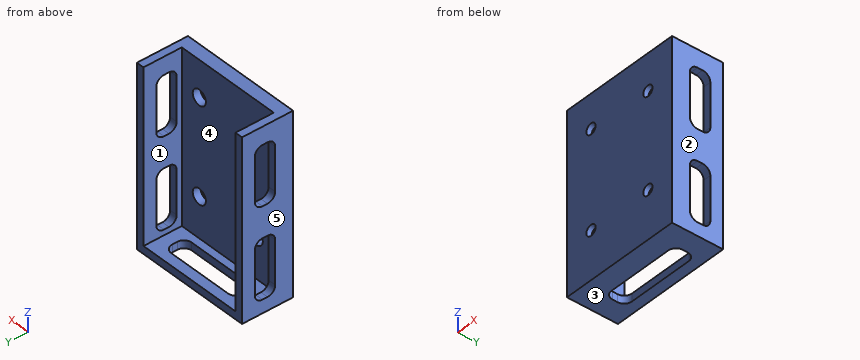
```python
from build123d import *

# Parameters (mm, degrees)
EXTRUDE_1_DEPTH     = 70
SKETCH_2_W          = 3
SKETCH_2_H          = 15
EXTRUDE_2_DEPTH     = 70
EXTRUDE_3_REACH     = 86.588
SKETCH_3_W          = 3
SKETCH_3_H          = 15
CUT_EXTRUDE_1_DEPTH = 87.22126548
CUT_EXTRUDE_2_DEPTH = 73.767483267
SKETCH_6_R          = 3
CUT_EXTRUDE_3_DEPTH = 3
SKETCH_7_R          = 2.1
CUT_EXTRUDE_4_DEPTH = 77.157731059


with BuildPart() as part:
    # 草图1 → 凸台-拉伸1 (new body)
    with BuildSketch(Plane.XY):
        Polygon((0, -15.16926567), (-24, -15.16926567), (-24, -10.16926567), (0, -10.16926567), (24, -10.16926567), (24, -15.16926567), align=None)
    extrude(amount=EXTRUDE_1_DEPTH)

    # 草图2 → 凸台-拉伸2 (add)
    with BuildSketch(Plane(origin=(0, 0, 0), x_dir=(-1, 0, 0), z_dir=(0, 0, -1))):
        with Locations((-22.5, -2.66926567)):
            Rectangle(SKETCH_2_W, SKETCH_2_H)
        with Locations((22.5, -2.66926567)):
            Rectangle(SKETCH_2_W, SKETCH_2_H)
    extrude(amount=-EXTRUDE_2_DEPTH)

    # 草图3 → 凸台-拉伸3 (add, up to next)
    with BuildSketch(Plane.ZY.offset(-21), mode=Mode.PRIVATE) as extrude_3_sk1:
        with Locations((1.5, -2.66926567)):
            Rectangle(SKETCH_3_W, SKETCH_3_H)
    extrude_3_tool1 = extrude(extrude_3_sk1.sketch, amount=EXTRUDE_3_REACH, mode=Mode.PRIVATE) - part.part
    add(extrude_3_tool1.solids().sort_by_distance((21, -2.669266, 1.5))[0])

    # 草图4 → 切除-拉伸1 (cut, through all)
    with BuildSketch(Plane.ZY.offset(24)):
        with BuildLine():
            Line((5.140274164, -3.16926567), (5.140274164, -5.16926567))
            ThreePointArc((5.140274164, -5.16926567), (6.018953821, -7.290586014), (8.140274164, -8.16926567))
            Line((8.140274164, -8.16926567), (25.140274164, -8.16926567))
            ThreePointArc((25.140274164, -8.16926567), (27.261594508, -7.290586014), (28.140274164, -5.16926567))
            Line((28.140274164, -5.16926567), (28.140274164, -3.16926567))
            ThreePointArc((28.140274164, -3.16926567), (27.261594508, -1.047945327), (25.140274164, -0.16926567))
            Line((25.140274164, -0.16926567), (8.140274164, -0.16926567))
            ThreePointArc((8.140274164, -0.16926567), (6.018953821, -1.047945327), (5.140274164, -3.16926567))
        make_face()
        with BuildLine():
            Line((40.140274164, -3.16926567), (40.140274164, -5.16926567))
            ThreePointArc((40.140274164, -5.16926567), (41.018953821, -7.290586014), (43.140274164, -8.16926567))
            Line((43.140274164, -8.16926567), (60.140274164, -8.16926567))
            ThreePointArc((60.140274164, -8.16926567), (62.261594508, -7.290586014), (63.140274164, -5.16926567))
            Line((63.140274164, -5.16926567), (63.140274164, -3.16926567))
            ThreePointArc((63.140274164, -3.16926567), (62.261594508, -1.047945327), (60.140274164, -0.16926567))
            Line((60.140274164, -0.16926567), (43.140274164, -0.16926567))
            ThreePointArc((43.140274164, -0.16926567), (41.018953821, -1.047945327), (40.140274164, -3.16926567))
        make_face()
    extrude(amount=-CUT_EXTRUDE_1_DEPTH, mode=Mode.SUBTRACT)

    # 草图5 → 切除-拉伸2 (cut, through all)
    with BuildSketch(Plane.XY.offset(3)):
        with BuildLine():
            Line((-13, 0.83073433), (13, 0.83073433))
            ThreePointArc((13, 0.83073433), (15.121320344, -0.047945327), (16, -2.16926567))
            Line((16, -2.16926567), (16, -4.16926567))
            ThreePointArc((16, -4.16926567), (15.121320344, -6.290586014), (13, -7.16926567))
            Line((13, -7.16926567), (-13, -7.16926567))
            ThreePointArc((-13, -7.16926567), (-15.121320344, -6.290586014), (-16, -4.16926567))
            Line((-16, -4.16926567), (-16, -2.16926567))
            ThreePointArc((-16, -2.16926567), (-15.121320344, -0.047945327), (-13, 0.83073433))
        make_face()
    extrude(amount=-CUT_EXTRUDE_2_DEPTH, mode=Mode.SUBTRACT)

    # 草图6 → 切除-拉伸3 (cut)
    with BuildSketch(Plane(origin=(0, -10.16926567, 0), x_dir=(1, 0, 0), z_dir=(0, 1, 0))):
        with Locations(Location((-13, -18.714712401, 0), (0, 0, 180))):
            Circle(SKETCH_6_R)
        with Locations(Location((13, -18.714712401, 0), (0, 0, 180))):
            Circle(SKETCH_6_R)
        with Locations(Location((-13, -56.714712401, 0), (0, 0, 180))):
            Circle(SKETCH_6_R)
        with Locations(Location((13, -55.851588753, 0), (0, 0, 180))):
            Circle(SKETCH_6_R)
    extrude(amount=-CUT_EXTRUDE_3_DEPTH, mode=Mode.SUBTRACT)

    # 草图7 → 切除-拉伸4 (cut, through all)
    with BuildSketch(Plane(origin=(0, -13.16926567, 0), x_dir=(1, 0, 0), z_dir=(0, 1, 0))):
        with Locations(Location((-13, -18.714712401, 0), (0, 0, 180))):
            Circle(SKETCH_7_R)
        with Locations(Location((13, -18.714712401, 0), (0, 0, 180))):
            Circle(SKETCH_7_R)
        with Locations(Location((13, -55.851588753, 0), (0, 0, 180))):
            Circle(SKETCH_7_R)
        with Locations(Location((-13, -56.714712401, 0), (0, 0, 180))):
            Circle(SKETCH_7_R)
    extrude(amount=-CUT_EXTRUDE_4_DEPTH, mode=Mode.SUBTRACT)


solid = part.part
```
Model file for the job. Use its own axes, mm. Face numbers are marked on the shaded views. A direction names the side the tool comes from. Give positions to 0.01 mm unless a question says otherwise; leave off trailing zeros. Write each loop counter-clockwise with the first axis right and the second up, starting at its lowest first coordinate (ties: lowest second). Pieces come first, ordered by that corner, then holes. Notation, with made-up numbers: (-25, 65.5) -> (5, 65.5) arc R17 ccw to (5, 82.5) -> close; hole circle Ø9 at (40, 27.25). An arc over 180 degrees is marked (long way). Use CSV: the item, a comma, the result in double quotes. Start each with the question number.
1) Two-plate mould, pull along X, no slides. Class the marked faces 3, 4 and 5: released by +X, released by -X, zero draft, split by the parting line, or undercut.
2) Pin check, flat tips, straight feed: P1, Ø1, axis at x = 18.5, y = -6, coming from the +Z side; P2, Ø1.5, axis at y = -1, z = 57.5, coming from the -X side. Stop position of each tip, or through.
3) Cut at A-A on x = 5. List the corners of the cut face in (y, z), plus the area to 3 significant figures.
4) Cut at C-C on y = -1.25. List the corners of the cut face in (x, z).
5) Drill centre lines: L1, parallel to Z at x = 13, y = -14.8; L2, parallel to Z at x = -13, y = -13.9; L3, parallel to X at y = 2, z = 7.5. Where is each one in solid material? Low to high.
6) Cut at D-D on z = 36.5. List the corners of the cut face in (x, y).
7) Tool access for the marked faces 1 and 2: list every direction of +Z, -Z, +X, -X, +Y, -Y with a clear straight run to the whole face (end or side of a thin tool).
8) Cut at B-B on z = 50. List the corners of the cut face in (x, y).
Final values:
1,face 3,"zero draft"
1,face 4,"undercut"
1,face 5,"released by -X"
2,P1,"stops at z = 3"
2,P2,"passes through"
3,outline,"(-15.17, 0) -> (-7.17, 0) -> (-7.17, 3) -> (-10.17, 3) -> (-10.17, 70) -> (-15.17, 70) -> close; (0.83, 0) -> (4.83, 0) -> (4.83, 3) -> (0.83, 3) -> close"
3,area,"371 mm2"
4,outline,"(-24, 0) -> (-15.86, 0) -> (-15.86, 3) -> (-21, 3) -> (-21, 5.83) -> (-24, 5.83) -> close; (-24, 27.45) -> (-21, 27.45) -> (-21, 40.83) -> (-24, 40.83) -> close; (-24, 62.45) -> (-21, 62.45) -> (-21, 70) -> (-24, 70) -> close; (15.86, 0) -> (24, 0) -> (24, 5.83) -> (21, 5.83) -> (21, 3) -> (15.86, 3) -> close; (21, 27.45) -> (24, 27.45) -> (24, 40.83) -> (21, 40.83) -> close; (21, 62.45) -> (24, 62.45) -> (24, 70) -> (21, 70) -> close"
5,L1,"z = 0 to 16.61, 20.81 to 53.75, 57.95 to 70"
5,L2,"z = 0 to 16.61, 20.81 to 54.61, 58.81 to 70"
5,L3,"x = -24 to -21, 21 to 24"
6,outline,"(-24, -15.17) -> (24, -15.17) -> (24, 4.83) -> (21, 4.83) -> (21, -10.17) -> (-21, -10.17) -> (-21, 4.83) -> (-24, 4.83) -> close"
7,face 1,"+Z, +Y"
7,face 2,"+Z, -Z, +X, +Y, -Y"
8,outline,"(-24, -15.17) -> (24, -15.17) -> (24, -8.17) -> (21, -8.17) -> (21, -10.17) -> (-21, -10.17) -> (-21, -8.17) -> (-24, -8.17) -> close; (-24, -0.17) -> (-21, -0.17) -> (-21, 4.83) -> (-24, 4.83) -> close; (21, -0.17) -> (24, -0.17) -> (24, 4.83) -> (21, 4.83) -> close"
